Verification items for the finished model (mm, model axes). Face numbers are marked on the shaded views. Coordinates: 2 decimals unless noted, no trailing zeros. Write each loop counter-clockwise with the first axis right and the second up, starting at its lowest first coordinate (ties: lowest second). Pieces come first, ordered by that corner, then holes. Notation, with made-up numbers: (51, 52) - (71, 52) arc R32 cw to (71, 86) - close; hole circle Ø5 at (84, 60). An arc over 180 degrees is marked (long way). Use CSV: the item, a comma, the result in double quotes. Start each with the question number.
```python
from build123d import *

# Parameters (mm, degrees)
BOSS_EXTRUDE2_DEPTH = 100
CUT_EXTRUDE1_DEPTH  = 99
EXTRUDE_THIN1_DEPTH = 5


with BuildPart() as part:
    # Sketch1 → Boss-Extrude2 (new body)
    with BuildSketch(Plane(origin=(0, 0, 0), x_dir=(0, 0, -1), z_dir=(1, 0, 0))):
        with BuildLine():
            Line((-55, 0), (55, 0))
            ThreePointArc((55, 0), (0, -55), (-55, 0))
        make_face()
    extrude(amount=BOSS_EXTRUDE2_DEPTH)

    # Sketch5 → Cut-Extrude1 (cut)
    with BuildSketch(Plane(origin=(100, 0, 0), x_dir=(0, 0, -1), z_dir=(1, 0, 0))):
        with BuildLine():
            Line((-54, 0), (54, 0))
            ThreePointArc((54, 0), (0, -54), (-54, 0))
        make_face()
    extrude(amount=-CUT_EXTRUDE1_DEPTH, mode=Mode.SUBTRACT)

    # Sketch6 → Extrude-Thin1 (add)
    with BuildSketch(Plane(origin=(1, 0, 0), x_dir=(0, 0, -1), z_dir=(1, 0, 0))):
        with BuildLine():
            ThreePointArc((47, 0), (0, -47), (-47, 0))
            Line((-47, 0), (-46, 0))
            ThreePointArc((-46, 0), (0, -46), (46, 0))
            Line((46, 0), (47, 0))
        make_face()
    extrude(amount=EXTRUDE_THIN1_DEPTH)


solid = part.part
```
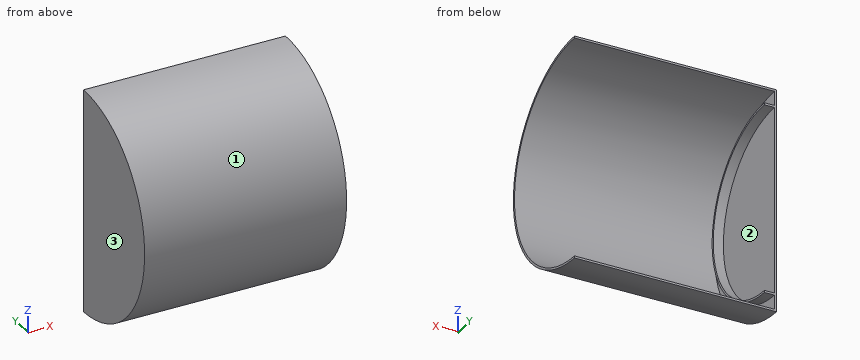
Q1. Gauge pin test, flat ends, axial feed: pin 1 (1 mm diameter, centred on x = 23, z = -40.5, fed in from -Y); pin 2 (1.5 mm diameter, centred on y = -23, z = 12.5, fed in from +X); pin 3 (10 mm diameter, centred on x = 59, y = -27, fed in from +Z). Record the tip position at first contact, or that the pin passes through.
Q2. Cross-section at C-C (y = -38). Record the cut outline in (x, z), plus the area to 3 significant figures.
Q3. Cross-section at D-D (z = 17). Record the cut outline in (x, y).
Q4. Release check for a two-part mould opening along Z. For the marked faces 1, 2 and 3 record: released by +Z, released by -Z, zero draft, split by the parting line, or undercut.
Q5. Scan lines: line 1 along X through (y, z) = (-49.5, 8); line 2 along Z through (x, y) = (70, -50); line 3 along X through (y, z) = (-6, -46.5). Record each from-to range of solid material in increasing order. Write a range as from..to.
Q6. Cross-section at B-B (x = 23.5). Record the cut outline in (y, z).
Q7. Cross-section at A-A (z = 0). Record the cut outline in (x, y), plus the area to 3 significant figures.
Reply:
1,pin 1,"y = -37.75"
1,pin 2,"x = 1"
1,pin 3,"z = 50.41"
2,outline,"(0, -39.76) - (100, -39.76) - (100, -38.37) - (1, -38.37) - (1, -27.66) - (6, -27.66) - (6, -25.92) - (1, -25.92) - (1, 25.92) - (6, 25.92) - (6, 27.66) - (1, 27.66) - (1, 38.37) - (100, 38.37) - (100, 39.76) - (0, 39.76) - close"
2,area,"373 mm^2"
3,outline,"(0, -52.31) - (100, -52.31) - (100, -51.25) - (1, -51.25) - (1, -43.82) - (6, -43.82) - (6, -42.74) - (1, -42.74) - (1, 0) - (0, 0) - close"
4,face 1,"split by the parting line"
4,face 2,"undercut"
4,face 3,"zero draft"
5,line 1,"0..1"
5,line 2,"-22.91..-20.4, 20.4..22.91"
5,line 3,"0..6"
6,outline,"(0, -55) - (0, -54) arc R54 cw to (0, 54) - (0, 55) arc R55 ccw to start"
7,outline,"(0, -55) - (100, -55) - (100, -54) - (1, -54) - (1, -47) - (6, -47) - (6, -46) - (1, -46) - (1, 0) - (0, 0) - close"
7,area,"159 mm^2"
